from build123d import *

# Parameters (mm, degrees)
BOSS_EXTRUDE1_DEPTH = 48
SKETCH2_W           = 0.5
SKETCH2_H           = 4.044844813
CUT_EXTRUDE1_DEPTH  = 2.25


with BuildPart() as part:
    # Sketch1 → Boss-Extrude1 (new body)
    with BuildSketch(Plane(origin=(0, 0, 0), x_dir=(0, 0, -1), z_dir=(1, 0, 0))):
        with BuildLine():
            Line((12.38, 0.625), (-12.38, 0.625))
            ThreePointArc((-12.38, 0.625), (-12.818406204, 0.443406204), (-13, 0.005))
            Line((-13, 0.005), (-13, -0.005))
            ThreePointArc((-13, -0.005), (-12.818406204, -0.443406204), (-12.38, -0.625))
            Line((-12.38, -0.625), (12.38, -0.625))
            ThreePointArc((12.38, -0.625), (12.818406204, -0.443406204), (13, -0.005))
            Line((13, -0.005), (13, 0.005))
            ThreePointArc((13, 0.005), (12.818406204, 0.443406204), (12.38, 0.625))
        make_face()
    extrude(amount=BOSS_EXTRUDE1_DEPTH)

    # Sketch2 → Cut-Extrude1 (cut, through all)
    with BuildSketch(Plane(origin=(0, 0.625, 0), x_dir=(1, 0, 0), z_dir=(0, 1, 0))):
        with BuildLine():
            ThreePointArc((12.25, 3.987468593), (12.5, -1), (12.75, 3.987468593))
            Line((12.75, 3.987468593), (12.75, 12.38))
            Line((12.75, 12.38), (12.25, 12.38))
            Line((12.25, 12.38), (12.25, 3.987468593))
        make_face()
        with BuildLine():
            Line((32.75, 12.38), (32.25, 12.38))
            Line((32.25, 12.38), (32.25, 3.987468593))
            ThreePointArc((32.25, 3.987468593), (32.5, -1), (32.75, 3.987468593))
            Line((32.75, 3.987468593), (32.75, 12.38))
        make_face()
        with Locations((12.5, 14.402422407)):
            Rectangle(SKETCH2_W, SKETCH2_H)
        with Locations((32.5, 14.402422407)):
            Rectangle(SKETCH2_W, SKETCH2_H)
    extrude(amount=-CUT_EXTRUDE1_DEPTH, mode=Mode.SUBTRACT)


solid = part.part
Input: part model. Units: mm. Frame: model coordinates. A direction names the side the tool comes from. Give positions to 0.01 mm unless a question says otherwise; leave off trailing zeros. Order: outer loops, then holes, each group sorted by start corner. A loop starts at its lowest first (then second) coordinate and runs counter-clockwise, first axis right, second up.
Q1. Section D-D on z = -1.5. Output: boundary loops of the cut face in (x, y) (3 decimals), and give its area (3 significant figures).
Checked values:
outline: (0, -0.625) - (10, -0.625) - (10, 0.625) - (0, 0.625) - close; (15, -0.625) - (30, -0.625) - (30, 0.625) - (15, 0.625) - close; (35, -0.625) - (48, -0.625) - (48, 0.625) - (35, 0.625) - close
area: 47.5 mm2
Q2. Set-up query: faces 5 (the flat face through (32.75, 0, -8)), 6 (the flat face through (24, -0.625, 0)). Return all of +Z, -Z, +X, -X, +Y, -Y with unobstructed straight access to the full face (end or side cutting, diameter ignored); none if empty.
Checked values:
face 5: -Z, +Y, -Y
face 6: +Z, -Z, +X, -X, -Y
Q3. Ray query, probe 1 along X at (y, z) = (-0.25, -1.5); probe 2 along Z at (x, y) = (31, -0.2); probe 3 along Z at (x, y) = (11, 0.25). Return the intervals inside material, ascending.
Checked values:
probe 1: x = 0 to 10, 15 to 30, 35 to 48
probe 2: z = -12.97 to -3.5, 0.5 to 12.97
probe 3: z = -12.95 to -3.5, 0.5 to 12.95
Q4. Section B-B on x = 34.5. Output: boundary loops of the cut face in (y, z) (3 decimals).
Checked values:
outline: (-0.625, -12.38) arc R0.62 ccw to (-0.005, -13) - (0.005, -13) arc R0.62 ccw to (0.625, -12.38) - (0.625, -3) - (-0.625, -3) - close; (-0.625, 0) - (0.625, 0) - (0.625, 12.38) arc R0.62 ccw to (0.005, 13) - (-0.005, 13) arc R0.62 ccw to (-0.625, 12.38) - close
Q5. Section A-A on z = -9.75. Output: boundary loops of the cut face in (x, y) (3 decimals), and give its area (4 significant figures).
Checked values:
outline: (0, -0.625) - (12.25, -0.625) - (12.25, 0.625) - (0, 0.625) - close; (12.75, -0.625) - (32.25, -0.625) - (32.25, 0.625) - (12.75, 0.625) - close; (32.75, -0.625) - (48, -0.625) - (48, 0.625) - (32.75, 0.625) - close
area: 58.75 mm2
Q6. Draft query along X for faces 1 (the flat face through (24, 0.625, 0)), 2 (the flat face through (0, 0, 0)), 3 (the cylindrical face through (12.4, 0, 1)), 4 (the flat face through (48, 0, 0)). Return one class per face: +X half, -X half, draft (parallel to the pull), parting line (faces both ways), or undercut.
Checked values:
face 1: draft
face 2: -X half
face 3: undercut
face 4: +X half
Q7. Section C-C on y = 0.3. Output: boundary loops of the cut face in (x, z), and give its area (3 significant figures).
Checked values:
outline: (0, -12.93) - (12.25, -12.93) - (12.25, -3.99) arc R2.5 cw (long way) to (12.75, -3.99) - (12.75, -12.93) - (32.25, -12.93) - (32.25, -3.99) arc R2.5 cw (long way) to (32.75, -3.99) - (32.75, -12.93) - (48, -12.93) - (48, 12.93) - (0, 12.93) - close
area: 1,190 mm2
